Autodesk Fusion 360 part; units mm, degrees
sketch "Sketch1" plane through (0, 0, 0) normal (0, 0, 1) x (1, 0, 0)
  line L0 (-5, 9.8) -> (5, 9.8)
  line L1 (5, 9.8) -> (5, 5)
  line L2 (5, 5) -> (10, 5)
  line L3 (10, 5) -> (10, 0)
  line L4 (5, -5) -> (-5, -5)
  line L5 (-10, 0) -> (-10, 5)
  line L6 (-10, 5) -> (-5, 5)
  line L7 (-5, 5) -> (-5, 9.8)
  line L8 (0, 0) -> (0, 9.8) construction
  line L9 (0, 0) -> (10, 0) construction
  line L10 (0, 0) -> (0, -5) construction
  line L11 (-5, 5) -> (-5, 0) construction
  line L12 (0, 0) -> (-5, 0) construction
  circle A0 centre (0, 0) radius 1.5
  line L13 (-10, -5) -> (-10, 0) construction
  line L14 (-5, -5) -> (-10, -5) construction
  arc A1 (-5, -5) -> (-10, 0) centre (-5, 0) ccw construction
  arc A2 (-10, 0) -> (-5, -5) centre (-5, 0) ccw
  line L15 (10, -5) -> (5, -5) construction
  line L16 (10, 0) -> (10, -5) construction
  arc A3 (10, 0) -> (5, -5) centre (5, 0) ccw construction
  arc A4 (5, -5) -> (10, 0) centre (5, 0) ccw
  point P0 (0, 9.8)
  point P1 (0, -5)
  point P2 (5, 0)
  dimension "d1" = 10
  dimension "d2" = 5
  dimension "d3" = 4.8
  dimension "d5" = 3
  dimension "d6" = 10
extrude "Extrude1" add sketch "Sketch1" along normal blind 4.8
Could you check a few things on this model? Use its own coordinates, in mm. A direction names the side the tool comes from. Round coordinates to 2 decimals unless told otherwise and drop trailing zeros. Order: outer loops, then holes, each group sorted by start corner. A loop starts at its lowest first (then second) coordinate and runs counter-clockwise, first axis right, second up.
Q1. Which directions (+Z, -Z, +X, -X, +Y, -Y) give clear straight access to the entire face, cutting with the end or side of a thin tool? Please do faces 1 (the face through (7, 5, 2)), 2 (the face through (-5, 7, 2)), 3 (the face through (0, 3, 0)).
Geometry says:
face 1: +Z, -Z, +X, +Y
face 2: +Z, -Z, -X, +Y
face 3: -Z, +X, -X, +Y, -Y
Q2. Imagine slicing it at B-B, the plane z = 0.6. List the corners of the cut face in (x, y) for me.
Geometry says:
outline: (-10, 0) arc R5 ccw to (-5, -5) - (5, -5) arc R5 ccw to (10, 0) - (10, 5) - (5, 5) - (5, 9.8) - (-5, 9.8) - (-5, 5) - (-10, 5) - close; hole circle Ø3 at (0, 0)
Q3. Imagine slicing it at A-A, the plane x = 0. List the corners of the cut face in (y, z) for me, then the cut area to 3 significant figures.
Geometry says:
outline: (-5, 0) - (-1.5, 0) - (-1.5, 4.8) - (-5, 4.8) - close; (1.5, 0) - (9.8, 0) - (9.8, 4.8) - (1.5, 4.8) - close
area: 56.6 mm2
Q4. Thinking about a two-plate mould opening in Y: for faces 4 (the face through (10, 3, 2)), 5 (the face through (-1.5, -0.07, 2.37)), 6 (the face through (-8, 5, 2)), 7 (the face through (-8, -4, 2)), which applies, released by +Y, released by -Y, zero draft, split by the parting line, or undercut?
Geometry says:
face 4: zero draft
face 5: undercut
face 6: released by +Y
face 7: released by -Y
Q5. Please list where these lines run through material, in increasing order: probe 1 along Y at (x, z) = (0, 1.9); probe 2 along X at (y, z) = (8.25, 1.5); probe 3 along X at (y, z) = (1, 3.55).
Geometry says:
probe 1: y = -5 to -1.5, 1.5 to 9.8
probe 2: x = -5 to 5
probe 3: x = -10 to -1.12, 1.12 to 10
Q6. Imagine slicing it at C-C, the plane y = -0.25. List the corners of the cut face in (x, z) for me, then the cut area to 3 significant figures.
Geometry says:
outline: (-9.99, 0) - (-1.48, 0) - (-1.48, 4.8) - (-9.99, 4.8) - close; (1.48, 0) - (9.99, 0) - (9.99, 4.8) - (1.48, 4.8) - close
area: 81.7 mm2
Q7. I'm going to push flat-ended pins straight in: P1, Ø2.5, axis at x = -7.5, z = 1.5, coming from the +Y side; P2, Ø1.5, axis at y = -1, z = 2.5, coming from the -X side; P3, Ø2.5, axis at y = 6.5, z = 3, coming from the +X side. Where does each tip first touch, or does it pass through?
Geometry says:
P1: stops at y = 5
P2: stops at x = -9.99
P3: stops at x = 5
Q8. Imagine slicing it at D-D, the plane x = 9. List the corners of the cut face in (y, z) for me, then the cut area to 3 significant figures.
Geometry says:
outline: (-3, 0) - (5, 0) - (5, 4.8) - (-3, 4.8) - close
area: 38.4 mm2
